Geometry check sheet. Reference: the model listing, model coordinates, mm. A direction names the side the tool comes from. Round coordinates to 2 decimals unless told otherwise and drop trailing zeros. Loops run counter-clockwise (first coordinate to the right, second up) from the corner with the lowest first, then second, coordinate; pieces in that order, holes last. Notation, with made-up numbers: (34.5, 37.25) - (71.5, 37.25) arc R31 cw to (71.5, 75.25) - close; hole circle Ø6 at (84.25, 87.5). An arc over 180 degrees is marked (long way). Answer as CSV lines item,"result". Start each with the question number.
1) Thickness scan on line 1 along Y through (x, z) = (-25, 3.25); line 2 along Y through (x, z) = (6, 11); line 3 along X through (y, z) = (-1.25, 11). Record the ranges inside material, lowest first.
2) Depth check by flat-ended pin: P1, Ø1.2, axis at x = -7, z = 7, coming from the +Y side; P2, Ø3.5, axis at y = -2, z = 10, coming from the -X side; P3, Ø1.5, axis at x = -23, z = 6, coming from the -Y side. Enter the tip coordinate at first touch or a pass-through.
3) Draft check along X on faces 4 (the flat face through (0, -2, 7)), 5 (the flat face through (11, 1, 7)), 6 (the flat face through (-38, -3, 7)), 7 (the flat face through (-60.369, -5.795, 7.395)). Enter one of: released by +X, released by -X, zero draft, split by the parting line, or undercut.
4) Cross-section at A-A on x = -20. Record the boundary of the cut face in (y, z), and give its area (3 significant figures).
5) Cross-section at B-B on y = -8. Record the boundary of the cut face in (x, z).
6) Access from +Z, -Z, +X, -X, +Y, -Y to the whole of each face (thin tool, end or side, straight path). Record for faces 1 (the flat face through (-6.7, -1.5, 7.4)), 2 (the flat face through (6, -3, 7)), 3 (the flat face through (-7, 0, 7)).
Autodesk Inventor part; units mm, degrees
ref_plane "YZ Plane" through (0, 0, 0) normal (1, 0, 0) x (0, 1, 0)
ref_plane "XZ Plane" through (0, 0, 0) normal (0, 1, 0) x (-1, 0, 0)
ref_plane "XY Plane" through (0, 0, 0) normal (0, 0, 1) x (1, 0, 0)
sketch "Эскиз1" plane through (0, 0, 0) normal (0, 0, 1) x (1, 0, 0)
  line L0 (0, 0) -> (1, 0)
  line L1 (9, 0) -> (9, -3) construction
  line L2 (9, -3) -> (3.5, -3) construction
  line L3 (0, -3) -> (0, 0)
  line L4 (0, -3) -> (-7.3989, -3)
  line L5 (-7.3989, -3) -> (-7.3989, -6) construction
  line L6 (-7.3989, -6) -> (0, -6)
  line L7 (0, -6) -> (0, -3) construction
  line L8 (0, -3) -> (2.5, -3) construction
  line L9 (2.5, -4) -> (2.5, -5)
  line L10 (1.5, -6) -> (0, -6)
  line L11 (0, -6) -> (0, -3) construction
  line L12 (-7.3989, -3) -> (-6, 0)
  line L13 (-7.3989, -3) -> (-13.5, -3) construction
  line L14 (-57.3989, -3) -> (-57.3989, -6) construction
  line L15 (-57.3989, -6) -> (-7.3989, -6)
  line L16 (-7.3989, -6) -> (-7.3989, -3) construction
  arc A0 (1.5, -6) -> (2.5, -5) centre (1.5, -5) ccw
  arc A1 (3.5, -3) -> (2.5, -4) centre (3.5, -4) ccw
  line L17 (-13.5, -3) -> (-17.5, -3) construction
  line L18 (0, 0) -> (1, 0)
  line L19 (9, 0) -> (8, 0) construction
  arc A2 (1, 0) -> (8, 0) centre (4.5, 9.3675) ccw construction
  line L20 (-57.3989, -3) -> (-59.5142, -3)
  line L21 (-59.5142, -3) -> (-62.1244, -11.5373)
  line L22 (-62.1244, -12.6534) -> (-58.474, -12.6534) construction
  line L23 (-58.474, -12.6534) -> (-58.474, -9.5163) construction
  line L24 (-58.474, -12.6534) -> (3.765, -31.6817)
  line L25 (3.765, -31.6817) -> (4.6422, -28.8128)
  line L26 (4.6422, -28.8128) -> (-58.474, -9.5163)
  line L27 (-58.474, -9.5163) -> (-58.474, -12.6534) construction
  line L28 (-57.3989, -6) -> (-57.3989, -3) construction
  line L29 (-58.474, -9.5163) -> (-57.3989, -6)
  line L30 (-13.5, -3) -> (-17.5, -3) construction
  line L31 (-17.5, -3) -> (-57.3989, -3)
  line L32 (1, 0) -> (8, 0) construction
  line L33 (8, 0) -> (9, 0) construction
  line L34 (-58.474, -12.6534) -> (-62.1244, -11.5373)
  line L35 (-62.1244, -11.5373) -> (-62.1244, -12.6534) construction
  line L36 (-6, 0) -> (-7.5, 0) construction
  line L37 (-7.5, 0) -> (-7.5, -3) construction
  line L38 (-7.5, 0) -> (-9.5, 0) construction
  line L39 (-7.5, 0) -> (-9.5, 0) construction
  line L40 (-9.5, 0) -> (-13.5, -3) construction
  line L41 (-13.5, -3) -> (-17.5, -3) construction
  spline S0 degree 3 poles (-7.5, 0) (-9.5, 0) (-13.5, -3) (-17.5, -3) knots 1 1 1 1 2 2 2 2
  line L42 (-7.5, 0) -> (-6, 0)
  line L43 (9, -3) -> (11, -3) construction
  line L44 (11, 0) -> (11, 1.5)
  line L45 (11, 1.5) -> (10.6727, 1.5)
  arc A3 (1, 0) -> (10.6727, 1.5) centre (4.5, 9.3675) ccw
  line L46 (3.5, -3) -> (8, -3)
  arc A4 (8, -3) -> (11, 0) centre (8, 0) ccw
  point P0 (2.5, -6)
  point P1 (0, -6)
  point P2 (2, -4)
  dimension "d0" = 9
  dimension "d1" = 3
  dimension "d3" = 3
  dimension "d4" = 2.5
  dimension "d5" = 3
  dimension "d6" = 50
  dimension "d9" = 1
  dimension "d10" = 1
  dimension "d11" = 4
  dimension "d13" = 3
  dimension "d14" = 1
  dimension "d15" = 1
  dimension "d16" = 10
  dimension "d17" = 3.6504
  dimension "d18" = 10
  dimension "d20" = 3
  dimension "d21" = 65.0828
  dimension "d25" = 3.677
  dimension "d26" = 66
  dimension "d27" = 90
  dimension "d28" = 107
  dimension "d29" = 65
  dimension "d30" = 6
  dimension "d31" = 3
  dimension "d32" = 1.5
  dimension "d33" = 6
  dimension "d34" = 2
  dimension "d37" = 2
  dimension "d38" = 4.5
  dimension "d39" = 3
  dimension "d40" = 2.9
extrude "Выдавливание1" add sketch "Эскиз1" along normal blind 15
sketch "Эскиз3" plane through (0, 0, 15) normal (0, 0, 1) x (1, 0, 0)
  line L0 (-57.3989, -6) -> (1.5, -6) construction
  arc A0 (1.5, -6) -> (2.5, -5) centre (1.5, -5) ccw construction
  arc A1 (3.5, -3) -> (2.5, -4) centre (3.5, -4) ccw construction
  line L1 (1, 0) -> (0, 0) construction
  line L2 (0, 0) -> (0, -3) construction
  line L3 (0, -3) -> (-7.3989, -3) construction
  line L4 (-7.3989, -3) -> (-6, 0) construction
  line L5 (-6, 0) -> (-7.5, 0) construction
  line L6 (-17.5, -3) -> (-59.5142, -3) construction
  line L7 (-59.5142, -3) -> (-62.1244, -11.5373) construction
  line L8 (-62.1244, -11.5373) -> (3.765, -31.6817) construction
  line L9 (3.765, -31.6817) -> (4.6422, -28.8128) construction
  line L10 (4.6422, -28.8128) -> (-58.474, -9.5163) construction
  line L11 (-58.474, -9.5163) -> (-57.3989, -6) construction
  line L12 (4.6422, -28.8128) -> (-58.474, -9.5163) construction
  line L13 (-58.474, -9.5163) -> (-61.2472, -8.6684)
  line L14 (-58.474, -9.5163) -> (8.3891, -25.5344)
  line L15 (8.3891, -25.5344) -> (5.592, -37.2821)
  line L16 (5.592, -37.2821) -> (-67.5523, -14.3814)
  line L17 (-67.5523, -14.3814) -> (-63.6325, -8.2805)
  line L18 (-63.6325, -8.2805) -> (-61.2472, -8.6684)
  line L19 (2.5, -5) -> (2.5, -4)
  line L20 (3.5, -3) -> (8, -3)
  arc A2 (8, -3) -> (11, 0) centre (8, 0) ccw
  line L21 (11, 0) -> (11, 1.5)
  line L22 (11, 1.5) -> (10.6727, 1.5)
  arc A3 (1, 0) -> (10.6727, 1.5) centre (4.5, 9.3675) ccw
extrude "Выдавливание2" cut sketch "Эскиз3" against normal blind 25
sketch "Эскиз4" plane through (0, 0, 15) normal (0, 0, 1) x (1, 0, 0)
  line L0 (-61.2472, -8.6684) -> (-58.474, -9.5163) construction
  line L1 (-58.474, -9.5163) -> (-57.3989, -6) construction
  line L2 (-57.3989, -6) -> (1.5, -6) construction
  arc A0 (1.5, -6) -> (2.5, -5) centre (1.5, -5) ccw construction
  line L3 (2.5, -5) -> (2.5, -4) construction
  arc A1 (3.5, -3) -> (2.5, -4) centre (3.5, -4) ccw construction
  line L4 (3.5, -3) -> (8, -3) construction
  arc A2 (8, -3) -> (11, 0) centre (8, 0) ccw construction
  line L5 (11, 0) -> (11, 1.5) construction
  line L6 (11, 1.5) -> (10.6727, 1.5) construction
  arc A3 (1, 0) -> (10.6727, 1.5) centre (4.5, 9.3675) ccw construction
  line L7 (1, 0) -> (0, 0) construction
  line L8 (0, 0) -> (0, -3) construction
  line L9 (0, -3) -> (-7.3989, -3) construction
  line L10 (-7.3989, -3) -> (-6, 0) construction
  line L11 (-6, 0) -> (-7.5, 0) construction
  line L12 (-17.5, -3) -> (-59.5142, -3) construction
  line L13 (-59.5142, -3) -> (-61.2472, -8.6684) construction
  arc A4 (1, 0) -> (10.6727, 1.5) centre (4.5, 9.3675) ccw construction
  line L14 (1, 0) -> (9, -3) construction
  line L15 (9, -3) -> (10.6727, 1.5) construction
  spline S0 degree 2 poles (1, 0) (9, -3) (10.6727, 1.5) knots 1 1 1 2 2 2 construction
  line L16 (1, 0) -> (10.6727, 1.5) construction
  line L17 (11, 1.5) -> (10.6727, 1.5)
  line L18 (11, 1.5) -> (10, 1.5)
  line L19 (1, 0) -> (9, -3) construction
  line L20 (9, -3) -> (10, 1.5) construction
  spline S1 degree 2 poles (1, 0) (9, -3) (10, 1.5) knots 1 1 1 2 2 2
  line L21 (11, 0) -> (11, 1.5)
  line L22 (11, 1.5) -> (10, 0.696)
  line L23 (10, 0.696) -> (9.7197, 0.6526)
  line L24 (1, 0) -> (10, 1.5)
  dimension "d43" = 1
extrude "Выдавливание3" add sketch "Эскиз4" against normal up to surface (15 mm away) contours L22 L23 S1 L18 L17
extrude "Выдавливание4" cut sketch "Эскиз4" against normal up to surface (15 mm away) contours S1 L24
properties part number "bat_lock03"
Answer block:
1,line 1,"y = -6 to -3"
1,line 2,"y = -3 to -1.19"
1,line 3,"x = -11.17 to -6.58, 0 to 10.73"
2,P1,"stops at y = 0"
2,P2,"stops at x = -59.74"
2,P3,"stops at y = -6"
3,face 4,"undercut"
3,face 5,"released by +X"
3,face 6,"zero draft"
3,face 7,"released by -X"
4,outline,"(-6, 0) - (-3, 0) - (-3, 15) - (-6, 15) - close"
4,area,"45.0 mm^2"
5,outline,"(-61.04, 0) - (-58.01, 0) - (-58.01, 15) - (-61.04, 15) - close"
6,face 1,"+Z, -Z"
6,face 2,"+Z, -Z, +X, -Y"
6,face 3,"+Z, -Z, -X, +Y"
